CAD build for the part. Positions are in the model's coordinates, mm. Round coordinates to 2 decimals unless told otherwise and drop trailing zeros. Write each loop counter-clockwise with the first axis right and the second up, starting at its lowest first coordinate (ties: lowest second). Pieces come first, ordered by that corner, then holes. Notation, with made-up numbers: M -16,7.5 L 35,7.5 A28 cw 35,45.5 Z; hole C 56.5,-35 d5. An arc over 180 degrees is marked long. Write each question's results on one line, items separated by ' | '. Start each with the question number.
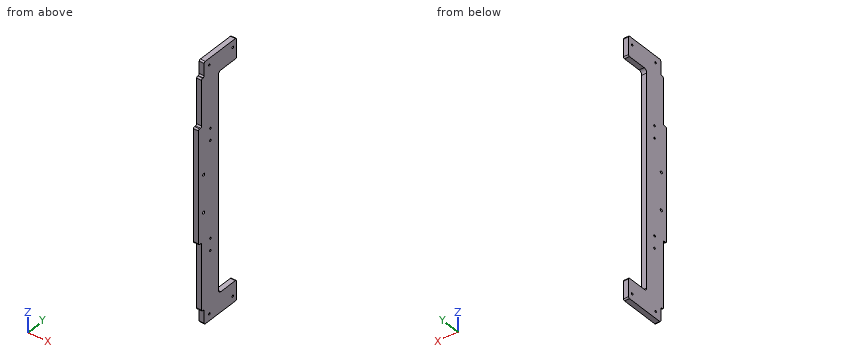
```python
from build123d import *

# Parameters (mm, degrees)
EXTRUDE_1_DEPTH     = 7.5
SKETCH_2_R          = 2
CUT_EXTRUDE_1_DEPTH = 8.5
SKETCH_9_W          = 78
SKETCH_9_H          = 32
SKETCH_9_W_2        = 103
EXTRUDE_3_DEPTH     = 7.5
SKETCH_11_W         = 30
SKETCH_11_H         = 35
EXTRUDE_4_DEPTH     = 7.5
SKETCH_10_R         = 1.5
CUT_EXTRUDE_6_DEPTH = 8.5
FILLET_1_R          = 2
FILLET_3_R          = 5
SKETCH_12_W         = 22
SKETCH_12_H         = 5
CUT_EXTRUDE_7_DEPTH = 8.5
FILLET_4_R          = 2
SKETCH_13_R         = 1.5
CUT_EXTRUDE_8_DEPTH = 8.5


with BuildPart() as part:
    # 草图1 → 凸台-拉伸1 (new body)
    with BuildSketch(Plane(origin=(0, 0, 0), x_dir=(0, 0, -1), z_dir=(1, 0, 0))):
        Polygon((0, 32), (0, 0), (15, 0), (15, -6), (185, -6), (185, 0), (205, 0), (205, 32), align=None)
    extrude(amount=EXTRUDE_1_DEPTH)

    # 草图2 → 切除-拉伸1 (cut, through all)
    with BuildSketch(Plane(origin=(7.5, 0, 0), x_dir=(0, 0, -1), z_dir=(1, 0, 0))):
        with Locations((86.95, 4)):
            Circle(SKETCH_2_R)
        with Locations((142.65, 4)):
            Circle(SKETCH_2_R)
    extrude(amount=-CUT_EXTRUDE_1_DEPTH, mode=Mode.SUBTRACT)

    # 草图9 → 凸台-拉伸3 (add)
    with BuildSketch(Plane(origin=(7.5, 0, 0), x_dir=(0, 0, -1), z_dir=(1, 0, 0))):
        with Locations((-39, 16)):
            Rectangle(SKETCH_9_W, SKETCH_9_H)
        with Locations((256.5, 16)):
            Rectangle(SKETCH_9_W_2, SKETCH_9_H)
    extrude(amount=-EXTRUDE_3_DEPTH)

    # 草图11 → 凸台-拉伸4 (add)
    with BuildSketch(Plane(origin=(7.5, 0, 0), x_dir=(0, 0, -1), z_dir=(1, 0, 0))):
        with Locations((-63, 49.5)):
            Rectangle(SKETCH_11_W, SKETCH_11_H)
        with Locations((293, 49.5)):
            Rectangle(SKETCH_11_W, SKETCH_11_H)
    extrude(amount=-EXTRUDE_4_DEPTH)

    # 草图10 → 切除-拉伸6 (cut, through all)
    with BuildSketch(Plane(origin=(7.5, 0, 0), x_dir=(0, 0, -1), z_dir=(1, 0, 0))):
        with Locations((-68, 15)):
            Circle(SKETCH_10_R)
        with Locations((298, 15)):
            Circle(SKETCH_10_R)
        with Locations((-68, 60)):
            Circle(SKETCH_10_R)
        with Locations((298, 60)):
            Circle(SKETCH_10_R)
    extrude(amount=-CUT_EXTRUDE_6_DEPTH, mode=Mode.SUBTRACT)

    # 圆角1
    fillet_1_edges = [part.edges().sort_by_distance(p)[0] for p in [
        (3.75, 0, -185),
        (3.75, -6, -185),
        (3.75, -6, -15),
        (3.75, 0, -15),
        (3.75, 0, 78),
        (3.75, 0, -308),
        (3.75, 67, 78),
        (3.75, 67, 48),
        (3.75, 67, -308),
        (3.75, 67, -278),
    ]]
    fillet(fillet_1_edges, radius=FILLET_1_R)

    # 圆角3
    fillet_3_edges = [part.edges().sort_by_distance(p)[0] for p in [
        (3.75, 32, 48),
        (3.75, 32, -278),
    ]]
    fillet(fillet_3_edges, radius=FILLET_3_R)

    # 草图12 → 切除-拉伸7 (cut, through all)
    with BuildSketch(Plane(origin=(7.5, 0, 0), x_dir=(0, 0, -1), z_dir=(1, 0, 0))):
        with Locations((-67, 2.5)):
            Rectangle(SKETCH_12_W, SKETCH_12_H)
        with Locations((297, 2.5)):
            Rectangle(SKETCH_12_W, SKETCH_12_H)
    extrude(amount=-CUT_EXTRUDE_7_DEPTH, mode=Mode.SUBTRACT)

    # 圆角4
    fillet_4_edges = [part.edges().sort_by_distance(p)[0] for p in [
        (3.75, 5, 78),
        (3.75, 5, 56),
        (3.75, 0, 56),
        (3.75, 5, -308),
        (3.75, 0, -286),
        (3.75, 5, -286),
    ]]
    fillet(fillet_4_edges, radius=FILLET_4_R)

    # 草图13 → 切除-拉伸8 (cut, through all)
    with BuildSketch(Plane(origin=(7.5, 0, 0), x_dir=(0, 0, -1), z_dir=(1, 0, 0))):
        with Locations((205.999999668, 17.000000039)):
            Circle(SKETCH_13_R)
        with Locations((187.999999668, 17.000000039)):
            Circle(SKETCH_13_R)
        with Locations((43.999999668, 17.000000039)):
            Circle(SKETCH_13_R)
        with Locations((25.999999668, 17.000000039)):
            Circle(SKETCH_13_R)
    extrude(amount=-CUT_EXTRUDE_8_DEPTH, mode=Mode.SUBTRACT)


solid = part.part
```
1) Saw through at C-C, the plane z = 27. Write the cut outline in (x, y), plus the area to 3 significant figures.
2) Saw through at A-A, the plane x = 2. State how many separate pieces and enclosed holes the cut face has, plus the area to 3 significant figures.
3) Wall check: line 1 along Y through (x, z) = (5, 68); line 2 along Z through (x, y) = (6.5, 50.5); line 3 along Y through (x, z) = (5.25, -188). Give the ranges that are in metal, low to high. Write a range as from..to.
4) Drop flat-ended pins along their axis: pin 1 Ø4 at (x, z) = (2.5, -94.5) entering from +Y; pin 2 Ø0.8 at (x, y) = (4, 2.5) entering from +Z; pin 3 Ø2 at (x, z) = (3, -255) entering from -Y. Give the stop position or say it passes through.
5) Saw through at B-B, the plane z = -173. Write the cut outline in (x, y).
Filled sheet:
1) outline: M 0,0 L 7.5,0 L 7.5,32 L 0,32 Z | area: 240 mm^2
2) separate pieces: 1 | enclosed holes: 10 | area: 15,200 mm^2
3) line 1: y = 5..13.5, 16.5..58.5, 61.5..67 | line 2: z = -308..-278, 48..78 | line 3: y = 0..15.5, 18.5..32
4) pin 1: stops at y = 32 | pin 2: stops at z = 56 | pin 3: stops at y = 0
5) outline: M 0,-6 L 7.5,-6 L 7.5,32 L 0,32 Z
